from build123d import *

# Parameters (mm, degrees)
F0_R        = 170
F0_R_2      = 148.8565935533
F1_DEPTH    = 50
F1_FACE_R   = 170
F1_FACE_R_2 = 148.8565935533
F2_R        = 200
F2_R_2      = 170
F3_DEPTH    = 1500
F4_SIZE     = 10
F6_DEPTH    = 600
F7_R        = 35
F8_DEPTH    = 600


with BuildPart() as f1:
    # F0 (on Top) → F1 (new body)
    with BuildSketch(Plane.XY):
        Circle(F0_R)
        Circle(F0_R_2, mode=Mode.SUBTRACT)
    extrude(amount=F1_DEPTH)

    # F1_face (on face) + F2 (on face) → F3 (join)
    with BuildSketch(Plane.XY.offset(50)):
        Circle(F1_FACE_R)
        Circle(F1_FACE_R_2, mode=Mode.SUBTRACT)
    with BuildSketch(Plane.XY.offset(50)):
        Circle(F2_R)
        Circle(F2_R_2, mode=Mode.SUBTRACT)
    extrude(amount=F3_DEPTH)

    # F4
    f4_edges = [f1.edges().sort_by_distance(p)[0] for p in [
        (-170, 0, 0),
        (-148.856594, 0, 0),
    ]]
    chamfer(f4_edges, length=F4_SIZE)

    # F5 (on face) → F6 (join)
    with BuildSketch(Plane(origin=(0, 0, 50), x_dir=(1, 0, 0), z_dir=(0, 0, -1))):
        with BuildLine():
            ThreePointArc((-32.6282500588, 197.3205445414), (-2.1909388027, 199.9879991079), (28.2975059651, 197.9880076069))
            ThreePointArc((28.2975059651, 197.9880076069), (-3.1678765377, 289.1624765686), (-32.6282500588, 197.3205445414))
        make_face()
    extrude(amount=-F6_DEPTH)

    # F7 (on face) → F8 (cut)
    with BuildSketch(Plane(origin=(0, 0, 50), x_dir=(1, 0, 0), z_dir=(0, 0, -1))):
        with Locations((-2.6110750469, 238.3378638878)):
            Circle(F7_R)
    extrude(amount=-F8_DEPTH, mode=Mode.SUBTRACT)


solid = f1.part
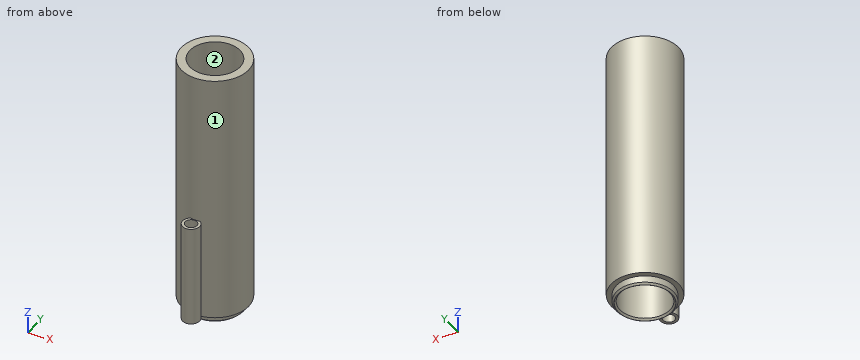
Geometry: final body of the model. Coordinates: model frame, mm. Face numbers are marked on the shaded views. Coordinates: 2 decimals unless noted, no trailing zeros. Order: outer loops, then holes, each group sorted by start corner. A loop starts at its lowest first (then second) coordinate and runs counter-clockwise, first axis right, second up.
(1) Material intervals for probe 1 along Y at (x, z) = (0, 568); probe 2 along Y at (x, z) = (0, 1240.5); probe 3 along X at (y, z) = (8, 666), sorted ascending.
(2) First-contact query: pin 1 (1 mm diameter, centred on x = 43, y = -180.5, fed in from -Z); pin 2 (2 mm diameter, centred on x = -24.5, z = 412.5, fed in from +Y); pin 3 (10 mm diameter, centred on x = -125.5, z = 589, fed in from -Y). Flat tips, straight axial feed; report the tip coordinate or a pass-through.
(3) Section query B-B (x = 0). Return the cut outline in (y, z), plus the area to 3 significant figures.
(4) Section query D-D (z = 255.5). Return the cut outline in (x, y).
(5) Section query A-A (y = 0). Return the cut outline in (x, z).
(6) Section query C-C (z = 1048.5). Return the cut outline in (x, y).
(7) Draft query along X for the marked faces 1 and 2. Return one class per face: pulls with the +X half, pulls with the -X half, needs draft (parallel to the pull), parting line crosses it, or undercut.
Solution:
1. probe 1: y = -289.1 to -273.24, -203.44 to -148.86, 148.86 to 200
1. probe 2: y = -200 to -148.86, 148.86 to 200
1. probe 3: x = -199.84 to -148.64, 148.64 to 199.84
2. pin 1: stops at z = 50
2. pin 2: stops at y = 198.61
2. pin 3: stops at y = -159.62
3. outline: (-289.1, 50) - (-273.24, 50) - (-273.24, 650) - (-289.1, 650) - close; (-203.44, 50) - (-170, 50) - (-170, 10) - (-160, 0) - (-158.86, 0) - (-148.86, 10) - (-148.86, 1550) - (-200, 1550) - (-200, 650) - (-203.44, 650) - close; (148.86, 10) - (158.86, 0) - (160, 0) - (170, 10) - (170, 50) - (200, 50) - (200, 1550) - (148.86, 1550) - close
3. area: 167,000 mm2
4. outline: (-32.63, -197.32) arc R50.83 ccw (long way) to (28.3, -197.99) arc R200 ccw (long way) to start; hole circle Ø297.71 at (0, 0); hole circle Ø70 at (-2.61, -238.34)
5. outline: (-200, 50) - (-170, 50) - (-170, 10) - (-160, 0) - (-158.86, 0) - (-148.86, 10) - (-148.86, 1550) - (-200, 1550) - close; (148.86, 10) - (158.86, 0) - (160, 0) - (170, 10) - (170, 50) - (200, 50) - (200, 1550) - (148.86, 1550) - close
6. outline: circle Ø400 at (0, 0); hole circle Ø297.71 at (0, 0)
7. face 1: parting line crosses it
7. face 2: undercut
